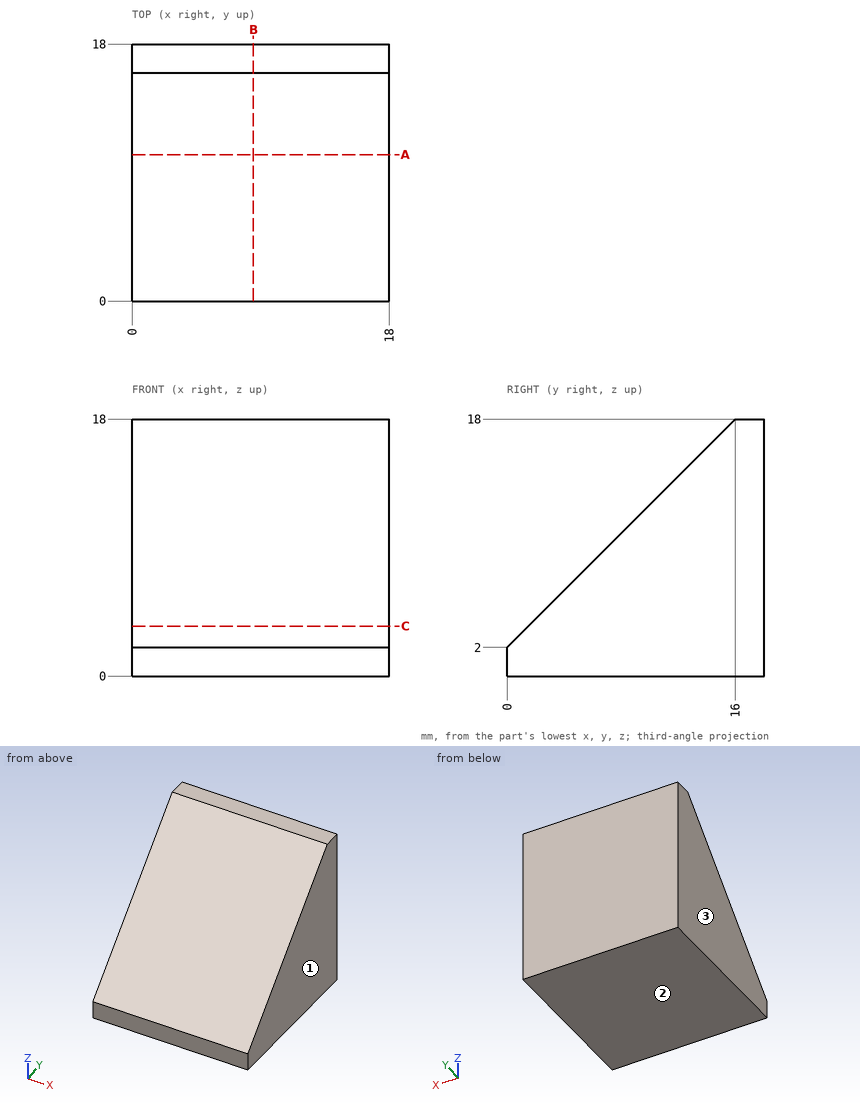
Input: dimensioned drawing with shaded views. Units: mm. Origin: part minimum x, y, z. Coordinates: 2 decimals unless noted, no trailing zeros. Loops run counter-clockwise (first coordinate to the right, second up) from the corner with the lowest first, then second, coordinate; pieces in that order, holes last.
Q1. Mould query, pull axis X, two halves, no side actions, for the marked faces 1, 2 and 3. Classes: +X half, -X half, draft (parallel to the pull), parting line (faces both ways), or undercut.
Results are:
face 1: +X half
face 2: draft
face 3: -X half
Q2. Line query: line 1 along Z through (x, y) = (17, 14); line 2 along Y through (x, z) = (15.5, 8.25); line 3 along Z through (x, y) = (15.5, 2.5). Output: solid intervals per line, ascending.
Results are:
line 1: z = 0 to 16
line 2: y = 6.25 to 18
line 3: z = 0 to 4.5
Q3. Section A-A, the plane y = 10.25. Return the cut outline in (x, z).
Results are:
outline: (0, 0) - (18, 0) - (18, 12.25) - (0, 12.25) - close
Q4. Section B-B, the plane x = 8.5. Return the cut outline in (y, z).
Results are:
outline: (0, 0) - (18, 0) - (18, 18) - (16, 18) - (0, 2) - close
Q5. Section C-C, the plane z = 3.5. Return the cut outline in (x, y).
Results are:
outline: (0, 1.5) - (18, 1.5) - (18, 18) - (0, 18) - close
Q6. Contact query for a flat-ended pin moving along its axis: pin 1 (4 mm diameter, centred on x = 2, z = 15, fed in from -Y). Output: stop coordinate, or through.
Results are:
pin 1: stops at y = 11
